from build123d import *

# Parameters (mm, degrees)
SKETCH1_R           = 15
BOSS_EXTRUDE1_DEPTH = 10
CUT_EXTRUDE1_DEPTH  = 24.452078799
SKETCH4_R           = 1.6
CUT_EXTRUDE2_DEPTH  = 10
CIRPATTERN2_COUNT   = 3


with BuildPart() as part:
    # Sketch1 → Boss-Extrude1 (new body)
    with BuildSketch(Plane(origin=(0, 0, 0), x_dir=(1, 0, 0), z_dir=(0, 1, 0))):
        with Locations(Location((0, 0, 0), (0, 0, 270))):
            Circle(SKETCH1_R)
    extrude(amount=BOSS_EXTRUDE1_DEPTH)

    # Sketch2 → Cut-Extrude1 (cut, through all)
    with BuildSketch(Plane(origin=(0, 10, 0), x_dir=(1, 0, 0), z_dir=(0, 1, 0))):
        Polygon((11.5, 0), (5.75, 9.959292144), (-5.75, 9.959292144), (-11.5, 0), (-5.75, -9.959292144), (5.75, -9.959292144), align=None)
    extrude(amount=-CUT_EXTRUDE1_DEPTH, mode=Mode.SUBTRACT)

    # Sketch4 → Cut-Extrude2 (cut)
    with BuildSketch(Plane(origin=(-12.990381057, 0, 7.5), x_dir=(0.5000000000000002, 0, 0.8660254037844386), z_dir=(-0.8660254037844385, 0, 0.5000000000000001))):
        with Locations((0, 5)):
            Circle(SKETCH4_R)
    cut_extrude2 = extrude(amount=-CUT_EXTRUDE2_DEPTH, mode=Mode.SUBTRACT)

    # CirPattern2: Cut-Extrude2 ×3 about axis
    cirpattern2_axis = Axis((0, 10, 0), (0, -1, 0))
    for i in range(1, CIRPATTERN2_COUNT):
        add(cut_extrude2.rotate(cirpattern2_axis, i * 360 / CIRPATTERN2_COUNT), mode=Mode.SUBTRACT)


solid = part.part
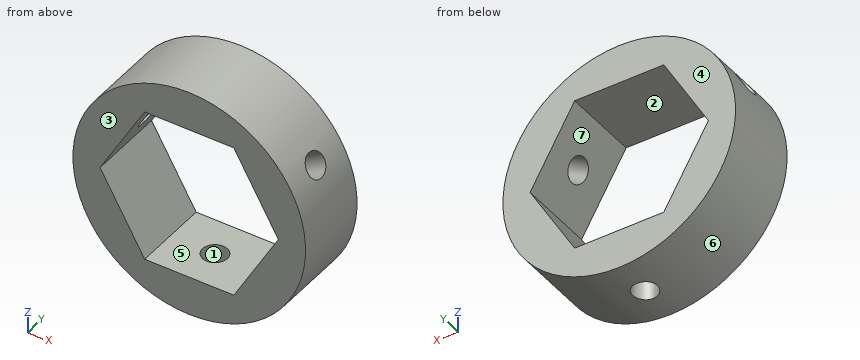
The listing builds one solid part. Answer for the finished solid, in the listing's coordinates (mm). Face numbers are marked on the shaded views. A direction names the side the tool comes from. Give positions to 0.01 mm unless a question says otherwise; leave off trailing zeros. Write each loop counter-clockwise with the first axis right and the second up, starting at its lowest first coordinate (ties: lowest second). Pieces come first, ordered by that corner, then holes.
1) Section B-B (z = 3) is taken. Write down the section's boundary in (x, y), and give its area (3 significant figures).
2) Section A-A (y = 1.5) is taken. Write down the section's boundary in (x, z).
3) Given P1, Ø3, axis at y = 4, z = 5, coming from the +X side; P2, Ø3, axis at x = 3, y = 5, coming from the +Z side; P3, Ø6, axis at x = -11, y = 4, coming from the -Z side, each flat-ended and moving along its own axis, determine where each tip first touches the part or whether it passes through.
4) Section D-D (y = 4.5) is taken. Write down the section's boundary in (x, z).
5) A tool of negligible diameter and unlimited length cuts with its end or side. For the marked faces 1, 2 and 3, from which of +Z, -Z, +X, -X, +Y, -Y can it reach the whole face along a straight path? Write none if from no direction.
6) Section C-C (x = 6.5) is taken. Write down the section's boundary in (y, z).
7) For a pull along X with two mould halves and no side action, classify the marked faces 4, 5, 6 and 7 as pulls with the +X half, pulls with the -X half, needs draft (parallel to the pull), parting line crosses it, or undercut.
8) Find the intervals of material crossed by L1, parallel to Y at x = 0, z = -12.5; L2, parallel to Z at x = -10.5, y = 6.25; L3, parallel to Z at x = 0.5, y = 9.25, in increasing order.
Response:
1. outline: (-14.7, 0) - (-9.77, 0) - (-9.77, 10) - (-14.7, 10) - close; (9.77, 0) - (14.7, 0) - (14.7, 10) - (9.77, 10) - close
1. area: 98.6 mm2
2. outline: circle Ø30 at (0, 0); hole (-11.5, 0) - (-5.75, -9.96) - (5.75, -9.96) - (11.5, 0) - (5.75, 9.96) - (-5.75, 9.96) - close
3. P1: stops at x = 14.59
3. P2: stops at z = 14.92
3. P3: stops at z = -12.69
4. outline: (-13.68, 6.15) arc R15 ccw to (-1.52, -14.92) - (-1.52, -9.96) - (-5.75, -9.96) - (-11.5, 0) - (-9.38, 3.66) - close; (-12.16, 8.78) - (-7.87, 6.3) - (-5.75, 9.96) - (5.75, 9.96) - (7.87, 6.3) - (12.16, 8.78) arc R15 ccw to start; (1.52, -14.92) arc R15 ccw to (13.68, 6.15) - (9.38, 3.66) - (11.5, 0) - (5.75, -9.96) - (1.52, -9.96) - close
5. face 1: -Z
5. face 2: +Y, -Y
5. face 3: +Z, -Z, +X, -X, -Y
6. outline: (0, -13.52) - (10, -13.52) - (10, -8.66) - (0, -8.66) - close; (0, 8.66) - (10, 8.66) - (10, 13.52) - (0, 13.52) - close
7. face 4: needs draft
7. face 5: undercut
7. face 6: parting line crosses it
7. face 7: undercut
8. L1: y = 0 to 3.4, 6.6 to 10
8. L2: z = -10.71 to -1.73, 1.73 to 4.91, 7.22 to 10.71
8. L3: z = -14.99 to -9.96, 9.96 to 14.99
